The model under review builds one solid part; all positions refer to its coordinate system, in mm. Face numbers are marked on the shaded views. A direction names the side the tool comes from. Give positions to 0.01 mm unless a question says otherwise; leave off trailing zeros. Loops run counter-clockwise (first coordinate to the right, second up) from the corner with the lowest first, then second, coordinate; pieces in that order, holes last. Notation, with made-up numbers: M 64,59 L 121,59 A19 ccw 121,87 Z; hole C -9,-39 d6. An arc over 180 degrees is marked long. Return JSON: item names as keys, results as strings.
Autodesk Inventor part; units mm, degrees
ref_plane "YZ Plane" through (0, 0, 0) normal (1, 0, 0) x (0, 1, 0)
ref_plane "XZ Plane" through (0, 0, 0) normal (0, 1, 0) x (-1, 0, 0)
ref_plane "XY Plane" through (0, 0, 0) normal (0, 0, 1) x (1, 0, 0)
sketch "Sketch1" plane through (0, 0, 0) normal (0, 1, 0) x (-1, 0, 0)
  line L0 (0, 0) -> (-16.51, 0)
  line L1 (-16.51, 0) -> (-16.51, -7.62)
  line L2 (-16.51, -7.62) -> (0, -7.62)
  line L3 (0, -7.62) -> (0, 0)
  line L4 (-8.255, 0) -> (-5.715, 0)
  line L5 (-5.715, 0) -> (-5.715, 6.35)
  line L6 (-5.715, 6.35) -> (-10.795, 6.35)
  line L7 (-10.795, 6.35) -> (-10.795, 0)
  line L8 (-5.715, -7.62) -> (-5.715, -8.89)
  line L9 (-5.715, -8.89) -> (-10.795, -8.89)
  line L10 (-10.795, -8.89) -> (-10.795, -7.62)
  line L11 (-10.795, 6.35) -> (-10.795, 3.81)
  line L12 (-10.795, 3.81) -> (-13.335, 3.81)
  line L13 (-13.335, 3.81) -> (-10.795, 6.35)
  line L14 (-5.715, 6.35) -> (-5.715, 3.81)
  line L15 (-5.715, 3.81) -> (-3.175, 3.81)
  line L16 (-3.175, 3.81) -> (-5.715, 6.35)
  point P0 (-8.255, -7.62)
  point P1 (0, -3.81)
  point P2 (-16.51, -3.81)
  dimension "d0" = 16.51
  dimension "d1" = 7.62
  dimension "d2" = 2.54
  dimension "d3" = 6.35
  dimension "d4" = 5.08
  dimension "d5" = 1.27
  dimension "d6" = 2.54
  dimension "d7" = 2.54
  dimension "d8" = 2.54
  dimension "d9" = 2.54
extrude "Extrusion1" add sketch "Sketch1" along normal blind 38.1
sketch "Sketch2" plane through (0, 38.1, 0) normal (0, 1, 0) x (1, 0, 0)
  line L0 (16.51, 0) -> (16.51, 7.62)
  line L1 (16.51, 3.81) -> (12.7, 3.81)
  line L2 (0, 7.62) -> (0, 0)
  circle A0 centre (12.7, 3.81) radius 1.016
  dimension "d12" = 3.81
  dimension "d14" = 2.032
extrude "Extrusion2" add sketch "Sketch2" along normal blind 1.27
sketch "Sketch3" plane through (0, 38.1, 0) normal (0, 1, 0) x (1, 0, 0)
  line L0 (0, 7.62) -> (0, 0)
  line L1 (0, 3.81) -> (3.81, 3.81)
  circle A0 centre (3.81, 3.81) radius 1.016
  dimension "d20" = 3.81
  dimension "d21" = 2.032
extrude "Extrusion3" add sketch "Sketch3" along normal blind 1.27
sketch "Sketch6" plane through (0, 38.1, 0) normal (0, 1, 0) x (1, 0, 0)
  line L0 (16.51, 0) -> (16.51, 7.62)
  line L1 (16.51, 3.81) -> (8.255, 3.81)
  circle A0 centre (8.255, 3.81) radius 1.397
  point P0 (0, 0)
  dimension "d24" = 8.255
  dimension "d25" = 2.794
hole "Hole1" at (8.255, 38.1, -3.81) at (8.255, 38.1, -3.81) direction (0, -1, 0) diameter 2.794 depth 11.43 tip angle 118
sketch "Sketch7" plane through (16.51, 0, 0) normal (1, 0, 0) x (0, 0, -1)
  line L0 (0, 0) -> (7.62, 0)
  line L1 (7.62, 0) -> (2.159, 0)
  line L2 (2.159, 0) -> (2.159, 10.16)
  line L3 (2.159, 10.16) -> (7.62, 10.16)
  line L4 (7.62, 10.16) -> (7.62, 0)
  dimension "d33" = 5.461
  dimension "d34" = 10.16
extrude "Extrusion4" add sketch "Sketch7" along normal blind 12.7
sketch "Sketch8" plane through (16.51, 0, -2.159) normal (0, 0, 1) x (1, 0, 0)
  line L0 (12.7, 0) -> (12.7, 10.16)
  line L1 (0, 10.16) -> (12.7, 10.16)
  line L2 (12.7, 0) -> (6.35, 0)
  line L3 (6.35, 0) -> (6.35, 10.16)
  line L4 (6.35, 10.16) -> (12.7, 10.16)
  line L5 (12.7, 10.16) -> (12.7, 0)
  point P0 (-16.51, 0)
extrude "Extrusion5" add sketch "Sketch8" along normal blind 22.479
sketch "Sketch11" plane through (16.51, 0, 20.32) normal (0, 0, 1) x (1, 0, 0)
  line L0 (12.7, 0) -> (12.7, 10.16)
  line L1 (12.7, 5.08) -> (9.525, 5.08)
  circle A0 centre (9.525, 5.08) radius 2.032
  point P0 (-16.51, 0)
  dimension "d41" = 3.175
  dimension "d42" = 4.064
extrude "Extrusion6" add sketch "Sketch11" along normal blind 5.08
sketch "Sketch12" plane through (26.035, 5.08, 25.4) normal (0, 0, 1) x (1, 0, 0)
  circle A0 centre (0, 0) radius 1.397
  point P0 (-26.035, -5.08)
  dimension "d45" = 2.794
hole "Hole2" at (26.035, 5.08, 25.4) direction (0, 0, -1) diameter 2.794 depth 12.7 tip angle 118
sketch "Sketch13" plane through (10.795, 0, -8.89) normal (0, 0, -1) x (-1, 0, 0)
  line L0 (0, 0) -> (0, 38.1)
  line L1 (0, 0) -> (5.08, 0)
  line L2 (0, 38.1) -> (5.08, 38.1)
  line L3 (5.08, 38.1) -> (5.08, 0)
  line L4 (5.08, 0) -> (0, 0)
  line L5 (0, 0) -> (0, 38.1)
  point P0 (10.795, 0)
extrude "Extrusion7" cut sketch "Sketch13" against normal blind 1.27
properties part number "Grab1"
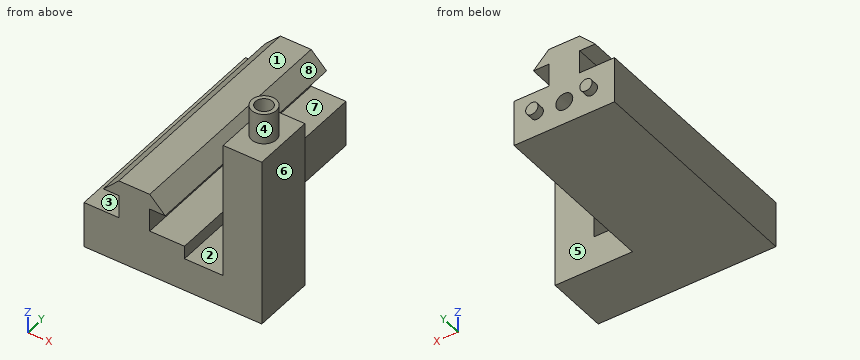
1) Consider section D-D on x = 16. Write out the cut boundary in (y, z).
From the geometry:
{"outline": "M 0,-7.62 L 38.1,-7.62 L 38.1,0 L 0,0 Z"}
2) Tool access review of the marked faces 1, 2, 3 and 4: name each direction out of +Z, -Z, +X, -X, +Y, -Y from which nothing blocks a thin tool from reaching the whole face with its end or side.
From the geometry:
{"face 1": "+Z, -X, +Y, -Y", "face 2": "+Z, +Y, -Y", "face 3": "-X, +Y, -Y", "face 4": "+Z"}
3) Wall thickness on L1, parallel to X at y = 5.08, z = 19; L2, parallel to Z at x = 22, y = 7; L3, parallel to Z at x = 7.5, y = 34.5: over which ranges is each line inside the solid? List them lowest first. Write a range as from..to.
From the geometry:
{"L1": "22.86..24.64, 27.43..29.21", "L2": "-7.62..-2.16", "L3": "-7.62..-4.99, -2.63..6.35"}
4) Consider section C-C on x = 3.81. Write out the cut boundary in (y, z) (3 decimals).
From the geometry:
{"outline": "M 0,-7.62 L 38.1,-7.62 L 38.1,-4.826 L 39.37,-4.826 L 39.37,-2.794 L 38.1,-2.794 L 38.1,0 L 0,0 Z; M 0,3.81 L 38.1,3.81 L 38.1,4.445 L 0,4.445 Z"}
5) The part is to be moulded in two halves that separate along X. For the marked faces 5, 6, 7 and 8, say which applies: released by +X, released by -X, zero draft, split by the parting line, or undercut.
From the geometry:
{"face 5": "zero draft", "face 6": "released by +X", "face 7": "undercut", "face 8": "undercut"}
6) Consider section B-B on y = 15. Write out the cut boundary in (x, z) (3 decimals), then the cut area to 3 significant figures.
From the geometry:
{"outline": "M 0,-7.62 L 16.51,-7.62 L 16.51,0 L 10.795,0 L 10.795,3.81 L 13.335,3.81 L 10.795,6.35 L 5.715,6.35 L 3.175,3.81 L 5.715,3.81 L 5.715,0 L 0,0 Z", "area": "165 mm²"}
7) Insertion check: pin 1 (4.5 mm diameter, centred on x = 2.5, y = 23, fed in from +Z) (3 decimals); pin 2 (5.5 mm diameter, centred on x = 8.5, y = 14, fed in from +Z); pin 3 (1.5 mm diameter, centred on y = 15.5, z = 7.5, fed in from -X); pin 4 (1.7 mm diameter, centred on x = 26.035, y = 5.08, fed in from +Z). Each pin has a flat end and moves straight along its axis. Give the tip position at first contact, or say it passes through.
From the geometry:
{"pin 1": "z = 5.385", "pin 2": "z = 6.35", "pin 3": "through", "pin 4": "z = 12.37"}
8) Consider section A-A on z = 4.5. Write out the cut boundary in (x, y) (3 decimals).
From the geometry:
{"outline": "M 3.865,0 L 12.645,0 L 12.645,38.1 L 3.865,38.1 Z; M 22.86,0 L 29.21,0 L 29.21,10.16 L 22.86,10.16 Z"}
